```python
from build123d import *

# Parameters (mm, degrees)
F0_W     = 150.591
F0_H     = 113.711
F0_R     = 7.5
F0_R_2   = 3.5
F1_DEPTH = 10
F2_R     = 2
F3_DEPTH = 17


with BuildPart() as f1:
    # F0 (on Top) → F1 (new body)
    with BuildSketch(Plane.XY):
        Rectangle(F0_W, F0_H)
        with Locations((-19.8485, -1.4755)):
            Circle(F0_R, mode=Mode.SUBTRACT)
        with Locations((41.5985, 23.9765)):
            Circle(F0_R_2, mode=Mode.SUBTRACT)
        with Locations((-19.8485, -1.4755)):
            Circle(F0_R)
        with Locations((41.5985, 23.9765)):
            Circle(F0_R_2)
    extrude(amount=F1_DEPTH)

    # F2
    f2_edges = [f1.edges().sort_by_distance(p)[0] for p in [
        (0, -56.8555, 10),
        (-75.2955, 0, 10),
        (0, 56.8555, 10),
        (75.2955, 0, 10),
    ]]
    fillet(f2_edges, radius=F2_R)

    # F0 (on Top) → F3 (join)
    with BuildSketch(Plane.XY):
        with Locations((-19.8485, -1.4755)):
            Circle(F0_R)
        with Locations((41.5985, 23.9765)):
            Circle(F0_R_2)
    extrude(amount=F3_DEPTH)


solid = f1.part
```
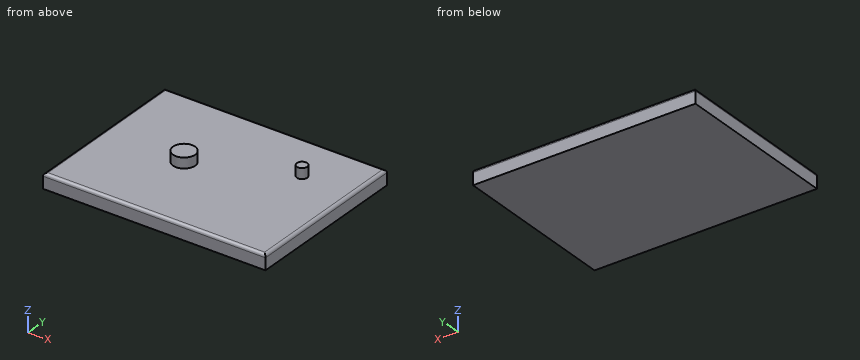
Input: part model. Units: mm. Frame: model coordinates. Coordinates: 2 decimals unless noted, no trailing zeros. Write each loop counter-clockwise with the first axis right and the second up, starting at its lowest first coordinate (ties: lowest second). Pieces come first, ordered by that corner, then holes. Notation, with made-up numbers: (70, 87) -> (118, 87) arc R24 cw to (118, 104) -> close; hole circle Ø5 at (-1.75, 82.5). An arc over 180 degrees is marked (long way). Answer as a JSON object with one key per item and string values.
1. First-contact query: P1, Ø2, axis at x = 25.5, y = 1.5, coming from the +Z side; P2, Ø4, axis at x = 44.5, y = 2, coming from the -Z side. Flat tips, straight axial feed; report the tip coordinate or a pass-through.
Result set:
{"P1": "stops at z = 10", "P2": "stops at z = 0"}
2. Section C-C on z = 12.5. Return the cut outline in (x, y), then the cut area to 3 significant figures.
Result set:
{"outline": "circle Ø15 at (-19.85, -1.48); circle Ø7 at (41.6, 23.98)", "area": "215 mm2"}
3. Material intervals for line 1 (Z direction, x = 50.5, y = -30); line 2 (X direction, y = 22, z = 9); line 3 (X direction, y = -42, z = 9.5), sorted ascending. Write a range as from..to.
Result set:
{"line 1": "z = 0..10", "line 2": "x = -75.03..75.03", "line 3": "x = -74.62..74.62"}
4. Section B-B on x = -9. Return the cut outline in (y, z), then the cut area to 3 significant figures.
Result set:
{"outline": "(-56.86, 0) -> (56.86, 0) -> (56.86, 8) arc R2 ccw to (54.86, 10) -> (-54.86, 10) arc R2 ccw to (-56.86, 8) -> close", "area": "1,140 mm2"}
5. Section A-A on y = 35. Return the cut outline in (x, z), then the cut area to 3 significant figures.
Result set:
{"outline": "(-75.3, 0) -> (75.3, 0) -> (75.3, 8) arc R2 ccw to (73.3, 10) -> (-73.3, 10) arc R2 ccw to (-75.3, 8) -> close", "area": "1,500 mm2"}
